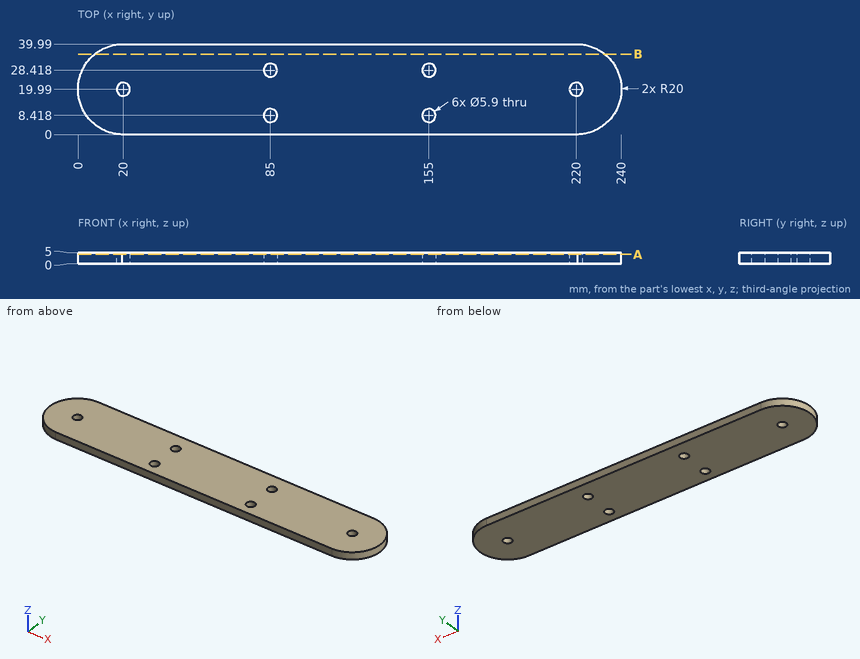
Drawing for the job (mm, zero at the part's lowest x, y, z). Give positions to 0.01 mm unless a question says otherwise; leave off trailing zeros. Write each loop counter-clockwise with the first axis right and the second up, starting at its lowest first coordinate (ties: lowest second). Pieces come first, ordered by that corner, then holes. Notation, with made-up numbers: (25.5, -33) -> (80.5, -33) arc R19 ccw to (80.5, -18) -> close; hole circle Ø2 at (77, 72). An arc over 180 degrees is marked (long way). Put each result on its own line as item: value. Start each with the question number.
Item 1: Cut at B-B (y = 35.5). List the corners of the cut face in (x, z), then the cut area to 3 significant figures.
Item 2: Cut at A-A (z = 4.2). List the corners of the cut face in (x, y).
Item 3: Wall check: L1, parallel to X at y = 20.5, z = 1.8 (1 decimal); L2, parallel to Y at x = 220.5, z = 3.4; L3, parallel to X at y = 11, z = 3.05 (1 decimal). Give the ranges that are in metal, low to high. Write a range as [from, to].
Item 4: Pin check, flat tips, straight feed: pin 1 Ø1 at (y, z) = (4.5, 0.5) entering from -X; pin 2 Ø5.5 at (x, y) = (85, 8.42) entering from -Z; pin 3 Ø1 at (y, z) = (32.5, 2) entering from -X. Stop position of each tip, or through.
Answer list:
1. outline: (7.37, 0) -> (232.63, 0) -> (232.63, 5) -> (7.37, 5) -> close
1. area: 1,130 mm2
2. outline: (19.37, 0) -> (220.63, 0) arc R20 ccw to (220, 39.99) -> (20, 39.99) arc R20 ccw to start; hole circle Ø5.9 at (20, 19.99); hole circle Ø5.9 at (85, 8.42); hole circle Ø5.9 at (85, 28.42); hole circle Ø5.9 at (155, 8.42); hole circle Ø5.9 at (155, 28.42); hole circle Ø5.9 at (220, 19.99)
3. L1: x = [0, 17.1], [22.9, 217.1], [222.9, 240]
3. L2: y = [0, 17.08], [22.9, 39.98]
3. L3: x = [2.1, 83.6], [86.4, 153.6], [156.4, 237.9]
4. pin 1: stops at x = 6.76
4. pin 2: passes through
4. pin 3: stops at x = 4.01
